Source: CAD feature listing. Evaluate the final solid. Frame: model axes, mm. Face numbers are marked on the shaded views. A direction names the side the tool comes from. Give positions to 0.01 mm unless a question says otherwise; leave off trailing zeros. Loops run counter-clockwise (first coordinate to the right, second up) from the corner with the lowest first, then second, coordinate; pieces in that order, holes last.
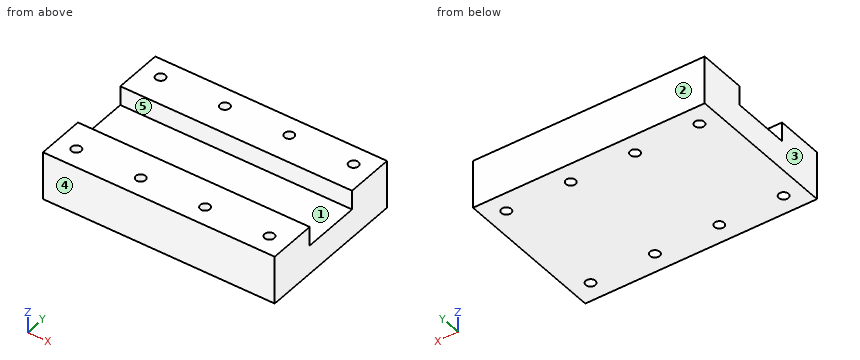
```python
from build123d import *

# Parameters (mm, degrees)
F0_W     = 76.2
F0_H     = 50.8
F0_R     = 1.5875
F1_DEPTH = 15.875
F2_W     = 76.2
F2_H     = 19.177
F3_DEPTH = 6.35


with BuildPart() as f1:
    # F0 (on Top) → F1 (new body)
    with BuildSketch(Plane.XY):
        Rectangle(F0_W, F0_H)
        with Locations((-31.75, -19.05)):
            Circle(F0_R, mode=Mode.SUBTRACT)
        with Locations((-10.583333, -19.05)):
            Circle(F0_R, mode=Mode.SUBTRACT)
        with Locations((10.583333, -19.05)):
            Circle(F0_R, mode=Mode.SUBTRACT)
        with Locations((31.75, -19.05)):
            Circle(F0_R, mode=Mode.SUBTRACT)
        with Locations((-31.75, 19.05)):
            Circle(F0_R, mode=Mode.SUBTRACT)
        with Locations((-10.583333, 19.05)):
            Circle(F0_R, mode=Mode.SUBTRACT)
        with Locations((10.583333, 19.05)):
            Circle(F0_R, mode=Mode.SUBTRACT)
        with Locations((31.75, 19.05)):
            Circle(F0_R, mode=Mode.SUBTRACT)
    extrude(amount=F1_DEPTH)

    # F2 (on face) → F3 (cut)
    with BuildSketch(Plane.XY.offset(15.875)):
        Rectangle(F2_W, F2_H)
    extrude(amount=-F3_DEPTH, mode=Mode.SUBTRACT)


solid = f1.part
```
(1) Section A-A, the plane z = 14.5. Count the separate pieces of the cut face and the enclosed holes in it, then the cut area to 3 significant figures.
A:
separate pieces: 2
enclosed holes: 8
area: 2,350 mm2
(2) Section B-B, the plane x = -31.75. Return the cut outline in (y, z) (1 decimal), then the cut area to 3 significant figures.
A:
outline: (-25.4, 0) - (-20.6, 0) - (-20.6, 15.9) - (-25.4, 15.9) - close; (-17.5, 0) - (17.5, 0) - (17.5, 15.9) - (9.6, 15.9) - (9.6, 9.5) - (-9.6, 9.5) - (-9.6, 15.9) - (-17.5, 15.9) - close; (20.6, 0) - (25.4, 0) - (25.4, 15.9) - (20.6, 15.9) - close
area: 584 mm2
(3) Section C-C, the plane y = -19.05. Return the cut outline in (x, z) (1 decimal), then the cut area to 3 significant figures.
A:
outline: (-38.1, 0) - (-33.3, 0) - (-33.3, 15.9) - (-38.1, 15.9) - close; (-30.2, 0) - (-12.2, 0) - (-12.2, 15.9) - (-30.2, 15.9) - close; (-9, 0) - (9, 0) - (9, 15.9) - (-9, 15.9) - close; (12.2, 0) - (30.2, 0) - (30.2, 15.9) - (12.2, 15.9) - close; (33.3, 0) - (38.1, 0) - (38.1, 15.9) - (33.3, 15.9) - close
area: 1,010 mm2
(4) Mould query, pull axis Y, two halves, no side actions, for the marked faces 3, 4 and 5. Classes: pulls with the +Y half, pulls with the -Y half, needs draft (parallel to the pull), parting line crosses it, or undercut.
A:
face 3: needs draft
face 4: pulls with the -Y half
face 5: undercut
(5) Reachability of the marked faces 1 and 2 from +Z, -Z, +X, -X, +Y, -Y: full face, straight path, thin tool, end or side. Return the list, or none.
A:
face 1: +Z, +X, -X
face 2: +Z, -Z, +X, -X, +Y
(6) Ray query, line 1 along Y through (x, z) = (-31.75, 4.5); line 2 along Y through (x, z) = (31.75, 12.5); line 3 along Y through (x, z) = (-4.5, 13.75). Return the intervals inside material, ascending.
A:
line 1: y = -25.4 to -20.64, -17.46 to 17.46, 20.64 to 25.4
line 2: y = -25.4 to -20.64, -17.46 to -9.59, 9.59 to 17.46, 20.64 to 25.4
line 3: y = -25.4 to -9.59, 9.59 to 25.4
